Geometry: final body of the model. Coordinates: model frame, mm. A direction names the side the tool comes from. Coordinates: 2 decimals unless noted, no trailing zeros. Loops run counter-clockwise (first coordinate to the right, second up) from the corner with the lowest first, then second, coordinate; pieces in that order, holes last. Notation, with made-up numbers: (6.25, -24) - (60.25, -24) arc R10 cw to (60.25, -12) - close; hole circle Ø9 at (77, 46.25). An arc over 180 degrees is marked (long way). Put each result on its own line as item: value. Start each with the question number.
1) Reachability of faces 1 (the cylindrical face through (-89.98, 2.46, 1.98)), 2 (the cylindrical face through (329.973, 2.465, -2.419)) from +Z, -Z, +X, -X, +Y, -Y: full face, straight path, thin tool, end or side. Return the list, or none.
2) Section B-B on z = 39. Output: boundary loops of the cut face in (x, y).
3) Draft query along Z for faces 3 (the flat face through (111, 5, -98)), 4 (the cylindrical face through (-109.973, 2.465, 2.419)), 5 (the cylindrical face through (309.98, 2.46, -1.98)). Return one class per face: +Z half, -Z half, draft (parallel to the pull), parting line (faces both ways), or undercut.
4) Material intervals for line 1 along Z through (x, y) = (148, 2.4); line 2 along Z through (x, y) = (16.5, 2.9); line 3 along X through (y, z) = (3.1, -50), sorted ascending. Write a range as from..to.
5) Section A-A on x = 104.5. Output: boundary loops of the cut face in (y, z).
6) Contact query for a flat-ended pin moving along its axis: pin 1 Ø3 at (x, y) = (-57, 4) entering from -Z. Output: stop coordinate, or through.
7) Section C-C on y = 2.3. Count the separate pieces of the cut face and the enclosed holes in it, and give its area (3 significant figures).
```python
from build123d import *

# Parameters (mm, degrees)
BOSS_EXTRUDE1_DEPTH          = 5
TAP_DRILL_FOR_M8X1_25_TAP1_D = 6.8


with BuildPart() as part:
    # Sketch1 → Boss-Extrude1 (new body)
    with BuildSketch(Plane(origin=(0, 0, 0), x_dir=(1, 0, 0), z_dir=(0, 1, 0))):
        with BuildLine():
            Line((0, 110), (220, 110))
            ThreePointArc((220, 110), (330, 0), (220, -110))
            Line((220, -110), (0, -110))
            ThreePointArc((0, -110), (-110, 0), (0, 110))
        make_face()
        with BuildLine():
            Line((0, 90), (220, 90))
            ThreePointArc((220, 90), (310, 0), (220, -90))
            Line((220, -90), (0, -90))
            ThreePointArc((0, -90), (-90, 0), (0, 90))
        make_face(mode=Mode.SUBTRACT)
    extrude(amount=BOSS_EXTRUDE1_DEPTH)

    # Tap Drill for M8x1.25 Tap1 (through all)
    with Locations(Plane(origin=(0, 5, 0), x_dir=(1, 0, 0), z_dir=(0, 1, 0))):
        with Locations((-86.602540378, -50), (0, -100), (220, 100), (-100, 0), (-86.602540378, 50), (0, 100), (74, 100), (148, 100), (290.710678119, 70.710678119), (320, 0), (290.710678119, -70.710678119), (220, -100), (148, -100), (74, -100)):
            Hole(TAP_DRILL_FOR_M8X1_25_TAP1_D / 2)


solid = part.part
```
Answer block:
1. face 1: +Y, -Y
1. face 2: +X, +Y, -Y
2. outline: (-102.85, 0) - (-81.11, 0) - (-81.11, 5) - (-102.85, 5) - close; (301.11, 0) - (322.85, 0) - (322.85, 5) - (301.11, 5) - close
3. face 3: draft
3. face 4: parting line
3. face 5: undercut
4. line 1: z = -110..-103.4, -96.6..-90, 90..96.6, 103.4..110
4. line 2: z = -110..-90, 90..110
4. line 3: x = -97.98..-90, -83.2..-74.83, 294.83..317.98
5. outline: (0, -110) - (5, -110) - (5, -90) - (0, -90) - close; (0, 90) - (5, 90) - (5, 110) - (0, 110) - close
6. pin 1: stops at z = -94.97
7. separate pieces: 1
7. enclosed holes: 15
7. area: 20,900 mm²
